Work out the finished part from the listing and answer in its coordinate system (mm). A direction names the side the tool comes from. Give positions to 0.01 mm unless a question says otherwise; leave off trailing zeros. Loops run counter-clockwise (first coordinate to the right, second up) from the corner with the lowest first, then second, coordinate; pieces in that order, holes last. Notation, with made-up numbers: (3.5, 38.25) - (55.5, 38.25) arc R31 ccw to (55.5, 65.25) - close; hole circle Ø10 at (-12.75, 56.5). An arc over 180 degrees is marked (long way). One line per question, with ' | ' between items.
from build123d import *

# Parameters (mm, degrees)
BOSS_EXTRUDE1_DEPTH = 2
SKETCH7_W           = 54.3
SKETCH7_H           = 30.2
SKETCH7_W_2         = 40.2
SKETCH7_H_2         = 20.2
BOSS_EXTRUDE3_DEPTH = 27
SKETCH8_W           = 40.2
SKETCH8_H           = 5
CUT_EXTRUDE2_DEPTH  = 27
CUT_EXTRUDE3_REACH  = 61.157
SKETCH9_W           = 25.2
SKETCH9_H           = 8.5
SKETCH10_R          = 0.95
CUT_EXTRUDE4_DEPTH  = 10
FILLET1_R           = 3
CUT_EXTRUDE5_REACH  = 59.459


with BuildPart() as part:
    # Sketch1 → Boss-Extrude1 (new body)
    with BuildSketch(Plane(origin=(0, 0, 0), x_dir=(1, 0, 0), z_dir=(0, 1, 0))):
        Polygon((-27.15, 10.1), (-27.15, -10.1), (-27.15, -15.1), (27.15, -15.1), (27.15, -10.1), (27.15, 10.1), (27.15, 15.1), (-27.15, 15.1), align=None)
    extrude(amount=BOSS_EXTRUDE1_DEPTH)

    # Sketch7 → Boss-Extrude3 (add)
    with BuildSketch(Plane(origin=(0, 2, 0), x_dir=(1, 0, 0), z_dir=(0, 1, 0))):
        Rectangle(SKETCH7_W, SKETCH7_H)
        Rectangle(SKETCH7_W_2, SKETCH7_H_2, mode=Mode.SUBTRACT)
    extrude(amount=BOSS_EXTRUDE3_DEPTH)

    # Sketch8 → Cut-Extrude2 (cut)
    with BuildSketch(Plane(origin=(0, 29, 0), x_dir=(1, 0, 0), z_dir=(0, 1, 0))):
        with Locations((0, -12.6)):
            Rectangle(SKETCH8_W, SKETCH8_H)
    extrude(amount=-CUT_EXTRUDE2_DEPTH, mode=Mode.SUBTRACT)

    # Sketch9 → Cut-Extrude3 (cut, up to next)
    with BuildSketch(Plane(origin=(-22.15, 0, 0), x_dir=(0, 0, -1), z_dir=(1, 0, 0)), mode=Mode.PRIVATE) as cut_extrude3_sk1:
        with Locations((-2.5, 6.25)):
            Rectangle(SKETCH9_W, SKETCH9_H)
    cut_extrude3_tool1 = extrude(cut_extrude3_sk1.sketch, amount=-CUT_EXTRUDE3_REACH, mode=Mode.PRIVATE) & part.part
    add(cut_extrude3_tool1.solids().sort_by_distance((-22.15, 6.25, 2.5))[0], mode=Mode.SUBTRACT)

    # Sketch10 → Cut-Extrude4 (cut)
    with BuildSketch(Plane(origin=(0, 29, 0), x_dir=(1, 0, 0), z_dir=(0, 1, 0))):
        with Locations(Location((-24.95, -5.425, 0), (0, 0, 270))):
            Circle(SKETCH10_R)
        with Locations(Location((-24.95, 5.425, 0), (0, 0, 90))):
            Circle(SKETCH10_R)
        with Locations(Location((24.95, -5.425, 0), (0, 0, 90))):
            Circle(SKETCH10_R)
        with Locations(Location((24.95, 5.425, 0), (0, 0, 270))):
            Circle(SKETCH10_R)
    extrude(amount=-CUT_EXTRUDE4_DEPTH, mode=Mode.SUBTRACT)

    # Fillet1
    fillet1_edges = [part.edges().sort_by_distance(p)[0] for p in [
        (-24.65, 10.5, 15.1),
    ]]
    fillet(fillet1_edges, radius=FILLET1_R)

    # Sketch12 → Cut-Extrude5 (cut, up to next)
    with BuildSketch(Plane(origin=(-20.1, 0, 0), x_dir=(0, 0, -1), z_dir=(1, 0, 0)), mode=Mode.PRIVATE) as cut_extrude5_sk1:
        with BuildLine():
            Line((-15.1, 2), (10.1, 2))
            Line((10.1, 2), (10.1, 10.5))
            Line((10.1, 10.5), (-12.1, 10.5))
            ThreePointArc((-12.1, 10.5), (-14.221320344, 11.378679656), (-15.1, 13.5))
            Line((-15.1, 13.5), (-15.1, 2))
        make_face()
    cut_extrude5_tool1 = extrude(cut_extrude5_sk1.sketch, amount=-CUT_EXTRUDE5_REACH, mode=Mode.PRIVATE) & part.part
    add(cut_extrude5_tool1.solids().sort_by_distance((-20.1, 6.293968, 2.606609))[0], mode=Mode.SUBTRACT)


solid = part.part
1. Find section D-D on x = -24.95. Write down the section's boundary in (y, z) (3 decimals).
Evaluation:
outline: (0, -15.1) - (29, -15.1) - (29, -6.375) - (19, -6.375) - (19, -4.475) - (29, -4.475) - (29, 4.475) - (19, 4.475) - (19, 6.375) - (29, 6.375) - (29, 15.1) - (13.5, 15.1) arc R3 ccw to (10.5, 12.1) - (10.5, -10.1) - (2, -10.1) - (2, 15.1) - (0, 15.1) - close
2. Flat-ended cylindrical pins translate along their axes: pin 1 (10 mm diameter, centred on x = -0.5, z = 10.5, fed in from +Y); pin 2 (0.6 mm diameter, centred on x = 25, z = 5.5, fed in from +Y); pin 3 (13.5 mm diameter, centred on x = -4.5, y = 17, fed in from +Z). Find the tip coordinate at first contact, or state that the pin passes through.
Evaluation:
pin 1: y = 2 | pin 2: y = 19 | pin 3: z = -10.1
3. Find section B-B on z = 1. Write down the section's boundary in (x, y).
Evaluation:
outline: (-27.15, 0) - (27.15, 0) - (27.15, 29) - (20.1, 29) - (20.1, 2) - (-27.15, 2) - close; (-27.15, 10.5) - (-20.1, 10.5) - (-20.1, 29) - (-27.15, 29) - close
4. Which of the six approach directions +Z, -Z, +X, -X, +Y, -Y give full straight-line access (tool end or side, diameter ignored) to faces 1 (the flat face through (-20.1, 20, 3)), 2 (the flat face through (-24, 10.5, 1)), 3 (the cylindrical face through (-24.01, 24.07, 5.3))?
Evaluation:
face 1: +Z, +Y | face 2: +Z, -X | face 3: +Y
5. Consider L1, parallel to X at y = 20, z = 3; L2, parallel to Y at x = -6, z = 6; L3, parallel to Y at x = -22, z = -1. Determine where each line is inside the solid, lowest interval first.
Evaluation:
L1: -27.15 to -20.1, 20.1 to 27.15 | L2: 0 to 2 | L3: 0 to 2, 10.5 to 29
6. Find section C-C on x = 24.95. Write down the section's boundary in (y, z) (3 decimals).
Evaluation:
outline: (0, -15.1) - (29, -15.1) - (29, -6.375) - (19, -6.375) - (19, -4.475) - (29, -4.475) - (29, 4.475) - (19, 4.475) - (19, 6.375) - (29, 6.375) - (29, 15.1) - (0, 15.1) - close
7. Find section A-A on y = 17. Write down the section's boundary in (x, z), then the cut area to 3 significant figures.
Evaluation:
outline: (-27.15, -15.1) - (27.15, -15.1) - (27.15, 15.1) - (20.1, 15.1) - (20.1, -10.1) - (-20.1, -10.1) - (-20.1, 15.1) - (-27.15, 15.1) - close | area: 627 mm2
8. Determine the mould class of faces 4 (the cylindrical face through (24.01, 24.07, 5.55)), 5 (the flat face through (27.15, 14, 0)), 6 (the flat face through (-3, 2, 3)) for opening direction X: +X half, -X half, draft (parallel to the pull), parting line (faces both ways), or undercut.
Evaluation:
face 4: undercut | face 5: +X half | face 6: draft
